```python
from build123d import *

# Parameters (mm, degrees)
SKETCH10_R         = 1.833087105
CUT_EXTRUDE2_DEPTH = 1.6129
CUT_EXTRUDE2_TAPER = 45
CUT_EXTRUDE1_DEPTH = 1.6129


with BuildPart() as part:
    # Sketch2 → Revolve1 (revolve)
    with BuildSketch(Plane(origin=(0, 0, 0), x_dir=(0, 0, -1), z_dir=(1, 0, 0))):
        with BuildLine():
            Line((-34.860484, 5.2197), (-31.6992, 2.471637744))
            ThreePointArc((-31.6992, 2.471637744), (-31.62608483, 2.428138789), (-31.542366229, 2.413))
            Line((-31.542366229, 2.413), (34.3296875, 2.413))
            Line((34.3296875, 2.413), (34.925, 1.8176875))
            Line((34.925, 1.8176875), (34.925, 0))
            Line((34.925, 0), (-34.925, 0))
            Line((-34.925, 0), (-34.925, 5.2197))
            Line((-34.925, 5.2197), (-34.860484, 5.2197))
        make_face()
    revolve(axis=Axis((0, 0, -34.925), (0, 0, 1)))

    # Sketch10 → Cut-Extrude2 (cut)
    with BuildSketch(Plane.XY.offset(34.925)):
        Circle(SKETCH10_R)
    extrude(amount=-CUT_EXTRUDE2_DEPTH, taper=CUT_EXTRUDE2_TAPER, mode=Mode.SUBTRACT)

    # Sketch9 → Cut-Extrude1 (cut)
    with BuildSketch(Plane.XY.offset(34.925)):
        Polygon((1.5875, -0.916543552), (1.5875, 0.916543552), (0, 1.833087105), (-1.5875, 0.916543552), (-1.5875, -0.916543552), (0, -1.833087105), align=None)
    extrude(amount=-CUT_EXTRUDE1_DEPTH, mode=Mode.SUBTRACT)


solid = part.part
```
Build history of the part. All positions in model axes, mm. A direction names the side the tool comes from. Coordinates: 2 decimals unless noted, no trailing zeros. Order: outer loops, then holes, each group sorted by start corner. A loop starts at its lowest first (then second) coordinate and runs counter-clockwise, first axis right, second up. Notation, with made-up numbers: (-35, 85.5) -> (-11, 85.5) arc R29 ccw to (-11, 116.5) -> close; hole circle Ø2 at (-39.75, -18). An arc over 180 degrees is marked (long way). Answer in a Markdown table with one row per item. Add a question column.
Q1. Band-saw the part on B-B, the plane z = -29.5. List the corners of the cut face in (x, y).
Q2. Mould opens along Y. For faces 1 (the face through (1.468, -1.915, -1.855)), 2 (the face through (2, 0, 34.925)), 3 (the face through (0.783, -1.381, 34.13)) say: +Y half, -Y half, draft (parallel to the pull), parting line (faces both ways), or undercut.
Q3. Drop flat-ended pins along their axis: pin 1 (4 mm diameter, centred on y = 1.5, z = 21, fed in from +X); pin 2 (2 mm diameter, centred on x = 1, z = 22, fed in from +Y); pin 3 (2 mm diameter, centred on x = 4, y = 3, fed in from -Z). Give the stop position or say it passes through.
Q4. Wall check: line 1 along Z through (x, y) = (0, 0.25) (3 decimals); line 2 along X through (y, z) = (0, -21); line 3 along Z through (x, y) = (2.25, -4.5) (3 decimals). Give the ranges that are in metal, low to high. Write a range as [from, to].
Q5. Which spindle directions (+Z, -Z, +X, -X, +Y, -Y) get a long thin tool onto all of the face, cutting with end or side? Do faces 4 (the face through (0, 0, 33.312)), 5 (the face through (0, 0, -34.925)). Say none if no direction does.
Answers follow:
| question | item | result |
|---|---|---|
| 1 | outline | circle Ø4.83 at (0, 0) |
| 2 | face 1 | parting line |
| 2 | face 2 | draft |
| 2 | face 3 | undercut |
| 3 | pin 1 | x = 2.41 |
| 3 | pin 2 | y = 2.41 |
| 3 | pin 3 | z = 33.46 |
| 4 | line 1 | [-34.925, 33.312] |
| 4 | line 2 | [-2.41, 2.41] |
| 4 | line 3 | [34.644, 34.925] |
| 5 | face 4 | +Z |
| 5 | face 5 | -Z, +X, -X, +Y, -Y |
